Geometry check sheet. Reference: the model listing, model coordinates, mm. Face numbers are marked on the shaded views. Round coordinates to 2 decimals unless told otherwise and drop trailing zeros. Write each loop counter-clockwise with the first axis right and the second up, starting at its lowest first coordinate (ties: lowest second). Pieces come first, ordered by that corner, then holes. Notation, with made-up numbers: M 49.25,72.5 L 94.25,72.5 A17 cw 94.25,94.5 Z; hole C 79,79.25 d9. An arc over 180 degrees is marked long. Answer in a Markdown table with one row per item. Add a question column.
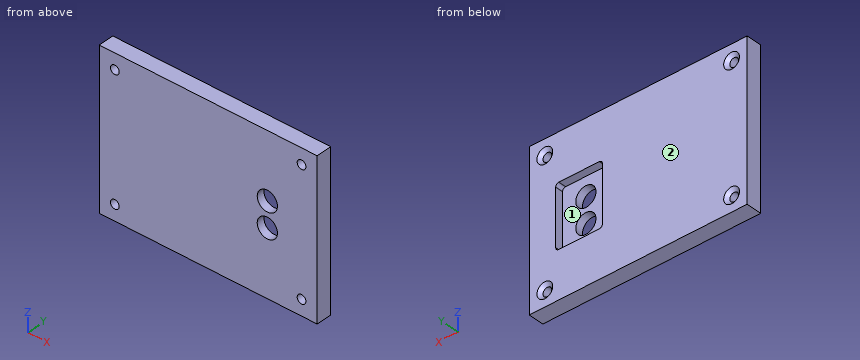
from build123d import *

# Parameters (mm, degrees)
SKETCH1_W                                           = 177.8
SKETCH1_H                                           = 127
BOSS_EXTRUDE1_DEPTH                                 = 12.7
CSK_FOR_1_4_FLAT_HEAD_MACHINE_SCREW_100_D           = 7.14248
CSK_FOR_1_4_FLAT_HEAD_MACHINE_SCREW_100_CSINK_D     = 12.8778
CSK_FOR_1_4_FLAT_HEAD_MACHINE_SCREW_100_CSINK_ANGLE = 100
SKETCH6_W                                           = 38.1
SKETCH6_H                                           = 50.8
CUT_EXTRUDE1_DEPTH                                  = 6.35
CUT_EXTRUDE2_REACH                                  = 111.434
SKETCH8_R                                           = 8.255
CUT_EXTRUDE3_REACH                                  = 111.434
SKETCH7_R                                           = 8.255
FILLET1_R                                           = 2.54


with BuildPart() as part:
    # Sketch1 → Boss-Extrude1 (new body)
    with BuildSketch(Plane(origin=(0, 0, 0), x_dir=(1, 0, 0), z_dir=(0, 1, 0))):
        Rectangle(SKETCH1_W, SKETCH1_H)
    extrude(amount=BOSS_EXTRUDE1_DEPTH)

    # CSK for 1/4 Flat Head Machine Screw (100)1 (through all)
    with Locations(Plane(origin=(0, 12.7, 0), x_dir=(1, 0, 0), z_dir=(0, 1, 0))):
        with Locations((-76.2, -50.8), (76.2, -50.8), (76.2, 50.8), (-76.2, 50.8)):
            CounterSinkHole(CSK_FOR_1_4_FLAT_HEAD_MACHINE_SCREW_100_D / 2, CSK_FOR_1_4_FLAT_HEAD_MACHINE_SCREW_100_CSINK_D / 2, counter_sink_angle=CSK_FOR_1_4_FLAT_HEAD_MACHINE_SCREW_100_CSINK_ANGLE)

    # Sketch6 → Cut-Extrude1 (cut)
    with BuildSketch(Plane(origin=(0, 12.7, 0), x_dir=(1, 0, 0), z_dir=(0, 1, 0))):
        with Locations((48.26, 0)):
            Rectangle(SKETCH6_W, SKETCH6_H)
    extrude(amount=-CUT_EXTRUDE1_DEPTH, mode=Mode.SUBTRACT)

    # Sketch8 → Cut-Extrude2 (cut, up to next)
    with BuildSketch(Plane(origin=(0, 6.35, 0), x_dir=(1, 0, 0), z_dir=(0, 1, 0)), mode=Mode.PRIVATE) as cut_extrude2_sk1:
        with Locations(Location((48.26, 10.16, 0), (0, 0, 270))):
            Circle(SKETCH8_R)
    cut_extrude2_tool1 = extrude(cut_extrude2_sk1.sketch, amount=-CUT_EXTRUDE2_REACH, mode=Mode.PRIVATE) & part.part
    add(cut_extrude2_tool1.solids().sort_by_distance((48.26, 6.35, -10.16))[0], mode=Mode.SUBTRACT)

    # Sketch7 → Cut-Extrude3 (cut, up to next)
    with BuildSketch(Plane(origin=(0, 6.35, 0), x_dir=(1, 0, 0), z_dir=(0, 1, 0)), mode=Mode.PRIVATE) as cut_extrude3_sk1:
        with Locations(Location((48.26, -10.16, 0), (0, 0, 270))):
            Circle(SKETCH7_R)
    cut_extrude3_tool1 = extrude(cut_extrude3_sk1.sketch, amount=-CUT_EXTRUDE3_REACH, mode=Mode.PRIVATE) & part.part
    add(cut_extrude3_tool1.solids().sort_by_distance((48.26, 6.35, 10.16))[0], mode=Mode.SUBTRACT)

    # Fillet1
    fillet1_edges = [part.edges().sort_by_distance(p)[0] for p in [
        (29.21, 9.525, -25.4),
        (67.31, 9.525, -25.4),
        (67.31, 9.525, 25.4),
        (29.21, 9.525, 25.4),
    ]]
    fillet(fillet1_edges, radius=FILLET1_R)


solid = part.part
Item 1: Section check C-C, the plane z = 10.16. Record the boundary of the cut face in (x, y) (3 decimals).
Item 2: Scan lines: probe 1 along Z at (x, y) = (-76.2, 3.5); probe 2 along X at (y, z) = (7, -50.8); probe 3 along X at (y, z) = (12.25, -51). Record each from-to range of solid material in increasing order. Write a range as from..to.
Item 3: Mould release check, pull along Z, two halves, no side actions. Record for the marked faces 1 and 2: +Z half, -Z half, draft (parallel to the pull), parting line (faces both ways), or undercut.
Item 4: Section check B-B, the plane z = -50.8. Record the boundary of the cut face in (x, y).
Item 5: Gauge pin test, flat end, axial feed: pin 1 Ø10 at (x, z) = (48.26, 10.16) entering from -Y. Record the tip position at first contact, or that the pin passes through.
Item 6: Section check A-A, the plane x = 48.26. Record the boundary of the cut face in (y, z) (3 decimals).
Result sheet:
| question | item | result |
|---|---|---|
| 1 | outline | M -88.9,0 L 40.005,0 L 40.005,6.35 L 29.21,6.35 L 29.21,12.7 L -88.9,12.7 Z; M 56.515,0 L 88.9,0 L 88.9,12.7 L 67.31,12.7 L 67.31,6.35 L 56.515,6.35 Z |
| 2 | probe 1 | z = -63.5..-54.37, -47.23..47.23, 54.37..63.5 |
| 2 | probe 2 | x = -88.9..-79.77, -72.63..72.63, 79.77..88.9 |
| 2 | probe 3 | x = -88.9..-82.1, -70.3..70.3, 82.1..88.9 |
| 3 | face 1 | undercut |
| 3 | face 2 | draft |
| 4 | outline | M -88.9,0 L -79.77,0 L -79.77,10.29 L -82.64,12.7 L -88.9,12.7 Z; M -72.63,0 L 72.63,0 L 72.63,10.29 L 69.76,12.7 L -69.76,12.7 L -72.63,10.29 Z; M 79.77,0 L 88.9,0 L 88.9,12.7 L 82.64,12.7 L 79.77,10.29 Z |
| 5 | pin 1 | passes through |
| 6 | outline | M 0,-63.5 L 12.7,-63.5 L 12.7,-25.4 L 6.35,-25.4 L 6.35,-18.415 L 0,-18.415 Z; M 0,-1.905 L 6.35,-1.905 L 6.35,1.905 L 0,1.905 Z; M 0,18.415 L 6.35,18.415 L 6.35,25.4 L 12.7,25.4 L 12.7,63.5 L 0,63.5 Z |
